Input: part model. Units: mm. Frame: model coordinates. Face numbers are marked on the shaded views. A direction names the side the tool comes from. Coordinates: 2 decimals unless noted, no trailing zeros. Write each loop counter-clockwise with the first axis right and the second up, starting at its lowest first coordinate (ties: lowest second). Pieces come first, ordered by that corner, then holes. Notation, with made-up numbers: (23.5, 76) - (27.5, 76) arc R28 cw to (27.5, 114) - close; hole circle Ø6 at (-25.75, -3). An arc over 180 degrees is marked (long way). Use a Markdown table: item, result. Add a question column.
Q1. Mould query, pull axis X, two halves, no side actions, for the marked faces 4, 5, 6 and 7. Classes: released by +X, released by -X, zero draft, split by the parting line, or undercut.
Q2. Material intervals for probe 1 along Z at (x, y) = (3.45, 5); probe 2 along X at (y, z) = (8.5, 0); probe 3 along X at (y, z) = (11, 13.5), sorted ascending. Write a range as from..to.
Q3. Section query B-B (z = 13.55). Return the cut outline in (x, y), then the cut area to 3 significant figures.
Q4. Pin query (flat end, axial travel): P1, Ø4, axis at y = 7, z = -5, coming from the +X side; P2, Ø2.5, axis at x = 25.55, z = 13.55, coming from the -Y side; P3, Ø1.5, axis at y = 1.5, z = 10, coming from the -X side; P4, Ø2, axis at x = -6.5, y = 4.5, coming from the +Z side. Return the tip coordinate at first contact, or that it passes through.
Q5. Section query C-C (z = -6). Return the cut outline in (x, y), then the cut area to 3 significant figures.
Q6. Section query A-A (x = 3.45). Return the cut outline in (y, z).
Q7. Set-up query: the marked faces 1, 2 and 3. Return all of +Z, -Z, +X, -X, +Y, -Y with unobstructed straight access to the full face (end or side cutting, diameter ignored); none if empty.
Q8. Section query D-D (y = 11). Return the cut outline in (x, z).
from build123d import *

# Parameters (mm, degrees)
BOSS_EXTRUDE1_DEPTH      = 20
BOSS_EXTRUDE1_DEPTH_BACK = 20
BOSS_EXTRUDE2_DEPTH      = 12
CUT_EXTRUDE1_DEPTH       = 53.704933355
CUT_EXTRUDE1_DEPTH_BACK  = 53.704933355
CUT_EXTRUDE2_DEPTH       = 53.704933355
CUT_EXTRUDE2_DEPTH_BACK  = 53.704933355
SKETCH7_R                = 1.5
CUT_EXTRUDE3_DEPTH       = 53.1110353


with BuildPart() as part:
    # Sketch1 → Boss-Extrude1 (new, two sides: drawn at the far end of the back side and taken through both)
    with BuildSketch(Plane(origin=(0, 0, 0), x_dir=(0, 1, 0), z_dir=(0, 0, 1)).offset(-BOSS_EXTRUDE1_DEPTH_BACK)):
        with BuildLine():
            ThreePointArc((0, -22.1), (7.6, -14.5), (0, -6.9))
            Line((0, -6.9), (0, 0))
            Line((0, 0), (12, 0))
            Line((12, 0), (12, -29))
            Line((12, -29), (0, -29))
            Line((0, -29), (0, -22.1))
        make_face()
    extrude(amount=BOSS_EXTRUDE1_DEPTH + BOSS_EXTRUDE1_DEPTH_BACK)

    # Sketch3 → Boss-Extrude2 (add)
    with BuildSketch(Plane(origin=(0, 12, 0), x_dir=(-1, 0, 0), z_dir=(0, 1, 0))):
        with BuildLine():
            Line((1.3, -7.1), (10.5, -7.1))
            ThreePointArc((10.5, -7.1), (17.6, 0), (10.5, 7.1))
            Line((10.5, 7.1), (0, 7.1))
            Line((0, 7.1), (0, -1.5))
            Line((0, -1.5), (6.684243194, -1.5))
            ThreePointArc((6.684243194, -1.5), (13.639126216, 2.637401486), (8.36458435, -3.5))
            Line((8.36458435, -3.5), (1.3, -3.5))
            Line((1.3, -3.5), (1.3, -7.1))
        make_face()
        with BuildLine():
            Line((-39.5, -7.1), (-29, -7.1))
            Line((-29, -7.1), (-29, 1.5))
            Line((-29, 1.5), (-35.684243194, 1.5))
            ThreePointArc((-35.684243194, 1.5), (-42.639126216, -2.637401486), (-37.36458435, 3.5))
            Line((-37.36458435, 3.5), (-30.3, 3.5))
            Line((-30.3, 3.5), (-30.3, 7.1))
            Line((-30.3, 7.1), (-39.5, 7.1))
            ThreePointArc((-39.5, 7.1), (-46.6, 0), (-39.5, -7.1))
        make_face()
    extrude(amount=-BOSS_EXTRUDE2_DEPTH)

    # Sketch4 → Cut-Extrude1 (cut, two sides: drawn at the far end of the back side and taken through both)
    with BuildSketch(Plane(origin=(0, 0, -1.5), x_dir=(1, 0, 0), z_dir=(0, 0, -1)).offset(-CUT_EXTRUDE1_DEPTH_BACK)):
        with BuildLine():
            ThreePointArc((-2.664243194, -6), (-4.164243194, -4.5), (-5.664243194, -6))
            Line((-5.664243194, -6), (-2.664243194, -6))
        make_face()
        with BuildLine():
            Line((-2.664243194, -6), (-5.664243194, -6))
            ThreePointArc((-5.664243194, -6), (-4.164243194, -7.5), (-2.664243194, -6))
        make_face()
    extrude(amount=CUT_EXTRUDE1_DEPTH + CUT_EXTRUDE1_DEPTH_BACK, mode=Mode.SUBTRACT)

    # Sketch5 → Cut-Extrude2 (cut, two sides: drawn at the far end of the back side and taken through both)
    with BuildSketch(Plane.XY.offset(1.5).offset(-CUT_EXTRUDE2_DEPTH_BACK)):
        with BuildLine():
            ThreePointArc((31.664243194, 6), (33.164243194, 4.5), (34.664243194, 6))
            Line((34.664243194, 6), (31.664243194, 6))
        make_face()
        with BuildLine():
            Line((31.664243194, 6), (34.664243194, 6))
            ThreePointArc((34.664243194, 6), (33.164243194, 7.5), (31.664243194, 6))
        make_face()
    extrude(amount=CUT_EXTRUDE2_DEPTH + CUT_EXTRUDE2_DEPTH_BACK, mode=Mode.SUBTRACT)

    # Sketch7 → Cut-Extrude3 (cut, through all)
    with BuildSketch(Plane.XZ):
        with Locations((3.45, 13.55)):
            Circle(SKETCH7_R)
        with Locations((25.55, -13.55)):
            Circle(SKETCH7_R)
        with Locations((25.55, 13.55)):
            Circle(SKETCH7_R)
        with Locations((3.45, -13.55)):
            Circle(SKETCH7_R)
    extrude(amount=-CUT_EXTRUDE3_DEPTH, mode=Mode.SUBTRACT)


solid = part.part
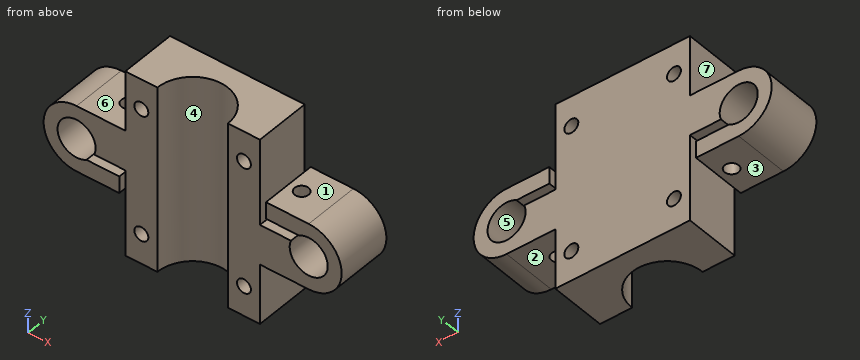
Values follow:
| question | item | result |
|---|---|---|
| 1 | face 4 | undercut |
| 1 | face 5 | undercut |
| 1 | face 6 | zero draft |
| 1 | face 7 | released by -X |
| 2 | probe 1 | -20..-15.05, -12.05..12.05, 15.05..20 |
| 2 | probe 2 | -17.6..-14.6, -6.4..35.4, 43.6..46.6 |
| 2 | probe 3 | 0..1.95, 4.95..24.05, 27.05..29 |
| 3 | outline | (0, 0) - (1.95, 0) - (1.95, 12) - (0, 12) - close; (4.95, 0) - (6.9, 0) arc R7.6 cw to (22.1, 0) - (24.05, 0) - (24.05, 12) - (4.95, 12) - close; (27.05, 0) - (29, 0) - (29, 12) - (27.05, 12) - close |
| 3 | area | 185 mm2 |
| 4 | P1 | x = 45.94 |
| 4 | P2 | through |
| 4 | P3 | x = 0 |
| 4 | P4 | z = 7.1 |
| 5 | outline | (-14.3, 0) - (-1.3, 0) - (-1.3, 12) - (-14.3, 12) - close; (0, 0) - (6.9, 0) arc R7.6 cw to (22.1, 0) - (43.3, 0) - (43.3, 12) - (0, 12) - close; hole circle Ø3 at (-4.16, 6); hole circle Ø3 at (33.16, 6) |
| 5 | area | 571 mm2 |
| 6 | outline | (0, -20) - (12, -20) - (12, -15.05) - (0, -15.05) - close; (0, -12.05) - (12, -12.05) - (12, 12.05) - (0, 12.05) - close; (0, 15.05) - (12, 15.05) - (12, 20) - (0, 20) - close |
| 7 | face 1 | +Z, +X, +Y, -Y |
| 7 | face 2 | -Z, +X, +Y, -Y |
| 7 | face 3 | -Z, -X, +Y, -Y |
| 8 | outline | (-10.5, -7.1) - (-1.3, -7.1) - (-1.3, -3.5) - (-8.36, -3.5) arc R4.1 cw (long way) to (-6.68, -1.5) - (0, -1.5) - (0, -20) - (29, -20) - (29, -7.1) - (39.5, -7.1) arc R7.1 ccw to (39.5, 7.1) - (30.3, 7.1) - (30.3, 3.5) - (37.36, 3.5) arc R4.1 cw (long way) to (35.68, 1.5) - (29, 1.5) - (29, 20) - (0, 20) - (0, 7.1) - (-10.5, 7.1) arc R7.1 ccw to start; hole circle Ø3 at (3.45, -13.55); hole circle Ø3 at (3.45, 13.55); hole circle Ø3 at (25.55, -13.55); hole circle Ø3 at (25.55, 13.55) |
